```python
from build123d import *
from OCP.BRepFilletAPI import BRepFilletAPI_MakeChamfer

# Parameters (mm, degrees)
EXTRUDE_1_DEPTH     = 6
EXTRUDE_1_DRAFT     = -6
CHAMFER_2_SIZE      = 1.123603797
CHAMFER_2_SIZE_2    = 1
SKETCH_3_3_R        = 1.55
CUT_EXTRUDE_1_DEPTH = 3.5
CHAMFER_3_SIZE      = 1
CHAMFER_3_SIZE_2    = 1.123603797


with BuildPart() as part:
    # 草图3 → 凸台-拉伸1 (with draft: the straight prism first)
    with BuildSketch(Plane.XY):
        with BuildLine():
            Line((-9.9049154, 123.558), (-9.9049154, -4.742307))
            ThreePointArc((-9.9049154, -4.742307), (-9.026235744, -6.863627344), (-6.9049154, -7.742307))
            Line((-6.9049154, -7.742307), (311.8950846, -7.742307))
            ThreePointArc((311.8950846, -7.742307), (314.016404944, -6.863627344), (314.8950846, -4.742307))
            Line((314.8950846, -4.742307), (314.8950846, 123.558))
            ThreePointArc((314.8950846, 123.558), (314.016404944, 125.679320344), (311.8950846, 126.558))
            Line((311.8950846, 126.558), (-6.9049154, 126.558))
            ThreePointArc((-6.9049154, 126.558), (-9.026235744, 125.679320344), (-9.9049154, 123.558))
        make_face()
        with BuildLine():
            Line((2.0950846, 116.558), (302.8950846, 116.558))
            ThreePointArc((302.8950846, 116.558), (305.016404944, 115.679320344), (305.8950846, 113.558))
            Line((305.8950846, 113.558), (305.8950846, 5.757693))
            ThreePointArc((305.8950846, 5.757693), (305.016404944, 3.636372656), (302.8950846, 2.757693))
            Line((302.8950846, 2.757693), (2.0950846, 2.757693))
            ThreePointArc((2.0950846, 2.757693), (-0.026235744, 3.636372656), (-0.9049154, 5.757693))
            Line((-0.9049154, 5.757693), (-0.9049154, 113.558))
            ThreePointArc((-0.9049154, 113.558), (-0.026235744, 115.679320344), (2.0950846, 116.558))
        make_face(mode=Mode.SUBTRACT)
    extrude(amount=-EXTRUDE_1_DEPTH)
    # 凸台-拉伸1: the draft: its side faces are tilted about the plane it starts from
    extrude_1_sides = [part.faces().sort_by_distance(p)[0] for p in [
        (152.4950846, 126.558, -3),
        (-9.026235744, 125.679320344, -3),
        (-9.9049154, 59.4078465, -3),
        (-9.026235744, -6.863627344, -3),
        (152.4950846, -7.742307, -3),
        (314.016404944, -6.863627344, -3),
        (314.8950846, 59.4078465, -3),
        (314.016404944, 125.679320344, -3),
        (-0.026235744, 115.679320344, -3),
        (152.4950846, 116.558, -3),
        (305.016404944, 115.679320344, -3),
        (305.8950846, 59.6578465, -3),
        (305.016404944, 3.636372656, -3),
        (152.4950846, 2.757693, -3),
        (-0.026235744, 3.636372656, -3),
        (-0.9049154, 59.6578465, -3),
    ]]
    draft(extrude_1_sides, Plane.XY, EXTRUDE_1_DRAFT)

    # 倒角2
    chamfer_2_edges_1 = [part.edges().sort_by_distance(p)[0] for p in [
        (-0.472155248, 116.125239848, -6),
    ]]
    chamfer_2_side_1 = [part.faces().sort_by_distance(p)[0] for p in [
        (-0.470676993, 116.123761593, -5.980109562),
    ]]
    chamfer_2_edges_2 = [part.edges().sort_by_distance(p)[0] for p in [
        (152.4950846, 117.188625412, -6),
    ]]
    chamfer_2_side_2 = [part.faces().sort_by_distance(p)[0] for p in [
        (152.4950846, 117.186534842, -5.980109562),
    ]]
    chamfer_2_edges_3 = [part.edges().sort_by_distance(p)[0] for p in [
        (305.462324448, 116.125239848, -6),
    ]]
    chamfer_2_side_3 = [part.faces().sort_by_distance(p)[0] for p in [
        (305.460846193, 116.123761593, -5.980109562),
    ]]
    chamfer_2_edges_4 = [part.edges().sort_by_distance(p)[0] for p in [
        (306.525710012, 59.6578465, -6),
    ]]
    chamfer_2_side_4 = [part.faces().sort_by_distance(p)[0] for p in [
        (306.523619442, 59.6578465, -5.980109562),
    ]]
    chamfer_2_edges_5 = [part.edges().sort_by_distance(p)[0] for p in [
        (305.462324448, 3.190453152, -6),
    ]]
    chamfer_2_side_5 = [part.faces().sort_by_distance(p)[0] for p in [
        (305.460846193, 3.191931407, -5.980109562),
    ]]
    chamfer_2_edges_6 = [part.edges().sort_by_distance(p)[0] for p in [
        (152.4950846, 2.127067588, -6),
    ]]
    chamfer_2_side_6 = [part.faces().sort_by_distance(p)[0] for p in [
        (152.4950846, 2.129158158, -5.980109562),
    ]]
    chamfer_2_edges_7 = [part.edges().sort_by_distance(p)[0] for p in [
        (-0.472155248, 3.190453152, -6),
    ]]
    chamfer_2_side_7 = [part.faces().sort_by_distance(p)[0] for p in [
        (-0.470676993, 3.191931407, -5.980109562),
    ]]
    chamfer_2_edges_8 = [part.edges().sort_by_distance(p)[0] for p in [
        (-1.535540812, 59.6578465, -6),
    ]]
    chamfer_2_side_8 = [part.faces().sort_by_distance(p)[0] for p in [
        (-1.533450242, 59.6578465, -5.980109562),
    ]]
    chamfer_2 = BRepFilletAPI_MakeChamfer(part.part.solid().wrapped)
    for e in chamfer_2_edges_1:
        chamfer_2.Add(CHAMFER_2_SIZE, CHAMFER_2_SIZE_2, e.wrapped, chamfer_2_side_1[0].wrapped)
    for e in chamfer_2_edges_2:
        chamfer_2.Add(CHAMFER_2_SIZE, CHAMFER_2_SIZE_2, e.wrapped, chamfer_2_side_2[0].wrapped)
    for e in chamfer_2_edges_3:
        chamfer_2.Add(CHAMFER_2_SIZE, CHAMFER_2_SIZE_2, e.wrapped, chamfer_2_side_3[0].wrapped)
    for e in chamfer_2_edges_4:
        chamfer_2.Add(CHAMFER_2_SIZE, CHAMFER_2_SIZE_2, e.wrapped, chamfer_2_side_4[0].wrapped)
    for e in chamfer_2_edges_5:
        chamfer_2.Add(CHAMFER_2_SIZE, CHAMFER_2_SIZE_2, e.wrapped, chamfer_2_side_5[0].wrapped)
    for e in chamfer_2_edges_6:
        chamfer_2.Add(CHAMFER_2_SIZE, CHAMFER_2_SIZE_2, e.wrapped, chamfer_2_side_6[0].wrapped)
    for e in chamfer_2_edges_7:
        chamfer_2.Add(CHAMFER_2_SIZE_2, CHAMFER_2_SIZE, e.wrapped, chamfer_2_side_7[0].wrapped)
    for e in chamfer_2_edges_8:
        chamfer_2.Add(CHAMFER_2_SIZE, CHAMFER_2_SIZE_2, e.wrapped, chamfer_2_side_8[0].wrapped)
    add(Compound.cast(chamfer_2.Shape()), mode=Mode.REPLACE)

    # 草图3<3> → 切除-拉伸1 (cut)
    with BuildSketch(Plane.XY):
        with Locations((-3.9049154, -3.742307)):
            Circle(SKETCH_3_3_R)
        with Locations((-3.9049154, 118.558)):
            Circle(SKETCH_3_3_R)
        with Locations((152.4955423, 118.558)):
            Circle(SKETCH_3_3_R)
        with Locations((308.896, 118.558)):
            Circle(SKETCH_3_3_R)
        with Locations((308.896, -3.742307)):
            Circle(SKETCH_3_3_R)
        with Locations((146.756, -3.742307)):
            Circle(SKETCH_3_3_R)
    extrude(amount=-CUT_EXTRUDE_1_DEPTH, mode=Mode.SUBTRACT)

    # 倒角3
    chamfer_3_edges_1 = [part.edges().sort_by_distance(p)[0] for p in [
        (152.4950846, 125.927374588, -6),
    ]]
    chamfer_3_side_1 = [part.faces().sort_by_distance(p)[0] for p in [
        (152.4950846, 125.907374588, -6),
    ]]
    chamfer_3_edges_2 = [part.edges().sort_by_distance(p)[0] for p in [
        (-8.580316239, 125.233400839, -6),
    ]]
    chamfer_3_side_2 = [part.faces().sort_by_distance(p)[0] for p in [
        (-8.566174103, 125.219258703, -6),
    ]]
    chamfer_3_edges_3 = [part.edges().sort_by_distance(p)[0] for p in [
        (-9.274289988, 59.4078465, -6),
    ]]
    chamfer_3_side_3 = [part.faces().sort_by_distance(p)[0] for p in [
        (-9.254289988, 59.4078465, -6),
    ]]
    chamfer_3_edges_4 = [part.edges().sort_by_distance(p)[0] for p in [
        (-8.580316239, -6.417707839, -6),
    ]]
    chamfer_3_side_4 = [part.faces().sort_by_distance(p)[0] for p in [
        (-8.566174103, -6.403565703, -6),
    ]]
    chamfer_3_edges_5 = [part.edges().sort_by_distance(p)[0] for p in [
        (152.4950846, -7.111681588, -6),
    ]]
    chamfer_3_side_5 = [part.faces().sort_by_distance(p)[0] for p in [
        (152.4950846, -7.091681588, -6),
    ]]
    chamfer_3_edges_6 = [part.edges().sort_by_distance(p)[0] for p in [
        (313.570485439, -6.417707839, -6),
    ]]
    chamfer_3_side_6 = [part.faces().sort_by_distance(p)[0] for p in [
        (313.556343303, -6.403565703, -6),
    ]]
    chamfer_3_edges_7 = [part.edges().sort_by_distance(p)[0] for p in [
        (314.264459188, 59.4078465, -6),
    ]]
    chamfer_3_side_7 = [part.faces().sort_by_distance(p)[0] for p in [
        (314.244459188, 59.4078465, -6),
    ]]
    chamfer_3_edges_8 = [part.edges().sort_by_distance(p)[0] for p in [
        (313.570485439, 125.233400839, -6),
    ]]
    chamfer_3_side_8 = [part.faces().sort_by_distance(p)[0] for p in [
        (313.556343303, 125.219258703, -6),
    ]]
    chamfer_3 = BRepFilletAPI_MakeChamfer(part.part.solid().wrapped)
    for e in chamfer_3_edges_1:
        chamfer_3.Add(CHAMFER_3_SIZE, CHAMFER_3_SIZE_2, e.wrapped, chamfer_3_side_1[0].wrapped)
    for e in chamfer_3_edges_2:
        chamfer_3.Add(CHAMFER_3_SIZE_2, CHAMFER_3_SIZE, e.wrapped, chamfer_3_side_2[0].wrapped)
    for e in chamfer_3_edges_3:
        chamfer_3.Add(CHAMFER_3_SIZE, CHAMFER_3_SIZE_2, e.wrapped, chamfer_3_side_3[0].wrapped)
    for e in chamfer_3_edges_4:
        chamfer_3.Add(CHAMFER_3_SIZE, CHAMFER_3_SIZE_2, e.wrapped, chamfer_3_side_4[0].wrapped)
    for e in chamfer_3_edges_5:
        chamfer_3.Add(CHAMFER_3_SIZE, CHAMFER_3_SIZE_2, e.wrapped, chamfer_3_side_5[0].wrapped)
    for e in chamfer_3_edges_6:
        chamfer_3.Add(CHAMFER_3_SIZE, CHAMFER_3_SIZE_2, e.wrapped, chamfer_3_side_6[0].wrapped)
    for e in chamfer_3_edges_7:
        chamfer_3.Add(CHAMFER_3_SIZE, CHAMFER_3_SIZE_2, e.wrapped, chamfer_3_side_7[0].wrapped)
    for e in chamfer_3_edges_8:
        chamfer_3.Add(CHAMFER_3_SIZE, CHAMFER_3_SIZE_2, e.wrapped, chamfer_3_side_8[0].wrapped)
    add(Compound.cast(chamfer_3.Shape()), mode=Mode.REPLACE)


solid = part.part
```
CAD build for the part. Positions are in the model's coordinates, mm. Round coordinates to 2 decimals unless told otherwise and drop trailing zeros. Write each loop counter-clockwise with the first axis right and the second up, starting at its lowest first coordinate (ties: lowest second). Pieces come first, ordered by that corner, then holes.
Item 1: Drill centre lines: L1, parallel to X at y = 84, z = -0.25; L2, parallel to Y at x = 219.5, z = -4.25; L3, parallel to Y at x = 66.5, z = -0.25. Where is each one in solid material? Low to high.
Filled in:
L1: x = -9.88 to -0.93, 305.92 to 314.87
L2: y = -7.3 to 2.31, 117 to 126.11
L3: y = -7.72 to 2.73, 116.58 to 126.53
Item 2: Band-saw the part on B-B on y = 60.5. Write the cut outline in (x, z), then the cut area to 3 significant figures.
Filled in:
outline: (-9.9, 0) - (-9.39, -4.88) - (-8.27, -6) - (-2.54, -6) - (-1.42, -4.88) - (-0.9, 0) - close; (305.9, 0) - (306.41, -4.88) - (307.53, -6) - (313.26, -6) - (314.38, -4.88) - (314.9, 0) - close
area: 98.2 mm2
Item 3: Band-saw the part on C-C on z = -2.5. Write the cut outline in (x, y).
Filled in:
outline: (-9.64, -4.74) arc R2.74 ccw to (-6.9, -7.48) - (311.9, -7.48) arc R2.74 ccw to (314.63, -4.74) - (314.63, 123.56) arc R2.74 ccw to (311.9, 126.3) - (-6.9, 126.3) arc R2.74 ccw to (-9.64, 123.56) - close; hole circle Ø3.1 at (-3.9, -3.74); hole circle Ø3.1 at (-3.9, 118.56); hole (-1.17, 5.76) arc R3.26 ccw to (2.1, 2.49) - (302.9, 2.49) arc R3.26 ccw to (306.16, 5.76) - (306.16, 113.56) arc R3.26 ccw to (302.9, 116.82) - (2.1, 116.82) arc R3.26 ccw to (-1.17, 113.56) - close; hole circle Ø3.1 at (146.76, -3.74); hole circle Ø3.1 at (152.5, 118.56); hole circle Ø3.1 at (308.9, -3.74); hole circle Ø3.1 at (308.9, 118.56)
Item 4: Drop flat-ended pins along their axis: pin 1 Ø0.9 at (x, y) = (146.5, -4.5) entering from +Z; pin 2 Ø1 at (x, z) = (239.5, -2.5) entering from -Y; pin 3 Ø3.5 at (x, y) = (-3.5, -3.5) entering from +Z; pin 4 Ø2 at (y, z) = (75.5, -5.5) entering from +X. Give the stop position or say it passes through.
Filled in:
pin 1: stops at z = -3.5
pin 2: stops at y = -7.53
pin 3: stops at z = 0
pin 4: stops at x = 314.42
Item 5: Band-saw the part on A-A on x = 112.5. Write the cut outline in (y, z).
Filled in:
outline: (-7.74, 0) - (-7.23, -4.88) - (-6.11, -6) - (1.13, -6) - (2.24, -4.88) - (2.76, 0) - close; (116.56, 0) - (117.07, -4.88) - (118.19, -6) - (124.93, -6) - (126.04, -4.88) - (126.56, 0) - close
